For this review, take the finished solid that the model builds, in its own axes (mm). Face numbers are marked on the shaded views. A direction names the side the tool comes from. Coordinates: 2 decimals unless noted, no trailing zeros. Order: outer loops, then holes, each group sorted by start corner. A loop starts at its lowest first (then second) coordinate and runs counter-clockwise, first axis right, second up. Notation, with made-up numbers: (58.5, 53.5) -> (88.5, 53.5) arc R16 cw to (88.5, 84.5) -> close; hole circle Ø11 at (-6.5, 75.5). An arc over 180 degrees is marked (long way). Write item = value, one per line. Start each with the question number.
1) Machinability: for the marked faces 1 and 2, which of the approach directions +Z, -Z, +X, -X, +Y, -Y give a long, thin tool a straight path to every point of the face, cutting with its end or side? Answer none if there is none.
2) Draft analysis for pull direction X (two halves, no side actions). For the marked faces 3, 4 and 5, state which applies: +X half, -X half, draft (parallel to the pull), parting line (faces both ways), or undercut.
3) Insertion check: pin 1 Ø6 at (x, z) = (-79, 7.5) entering from -Y; pin 2 Ø4 at (x, z) = (-54, 30) entering from +Y; pin 3 Ø6 at (y, z) = (10, 43) entering from -X; pin 4 Ø5 at (x, y) = (31, 14.5) entering from -Z. Each pin has a flat end and moves straight along its axis. Give the tip position at first contact, or say it passes through.
4) Wall thickness on probe 1 along Y at (x, z) = (-70, 32.5); probe 2 along Z at (x, y) = (-20.5, 45.5); probe 3 along X at (y, z) = (2, 4): over which ranges is each line inside the solid? List them lowest first. Write a range as [from, to].
5) Consider section A-A on x = 54. Give the boundary of the cut face in (y, z).
6) Consider section D-D on y = -23. Give the boundary of the cut face in (x, z), and give its area (3 significant figures).
7) Consider section C-C on z = 4.5. Give the boundary of the cut face in (x, y).
8) Consider section B-B on y = -10. Give the boundary of the cut face in (x, z), and give its area (3 significant figures).
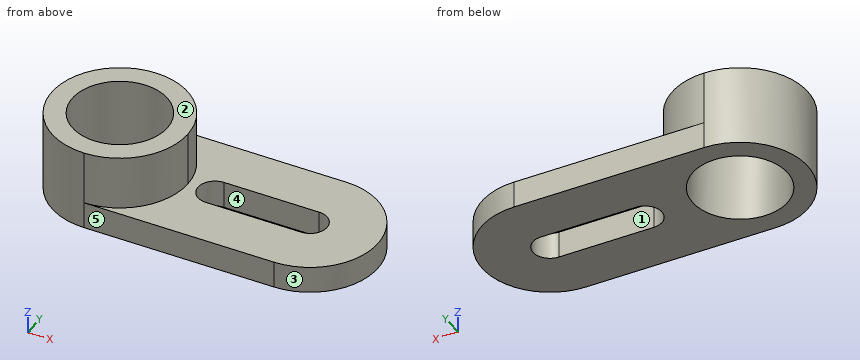
from build123d import *

# Parameters (mm, degrees)
F0_R     = 35
F1_DEPTH = 20
F2_DEPTH = 60


with BuildPart() as f1:
    # F0 (on Top) → F1 (new body)
    with BuildSketch(Plane.XY):
        with BuildLine():
            ThreePointArc((-70, -50), (-34.644661, -35.355339), (-20, 0))
            ThreePointArc((-20, 0), (-34.644661, 35.355339), (-70, 50))
            ThreePointArc((-70, 50), (-120, 0), (-70, -50))
        make_face()
        with Locations((-70, 0)):
            Circle(F0_R, mode=Mode.SUBTRACT)
        with BuildLine():
            ThreePointArc((-70, 50), (-34.644661, 35.355339), (-20, 0))
            ThreePointArc((-20, 0), (-34.644661, -35.355339), (-70, -50))
            Line((-70, -50), (70, -50))
            ThreePointArc((70, -50), (120, 0), (70, 50))
            Line((70, 50), (-70, 50))
        make_face()
        with BuildLine():
            Line((70, -12.5), (0, -12.5))
            ThreePointArc((0, -12.5), (-12.5, 0), (0, 12.5))
            Line((0, 12.5), (70, 12.5))
            ThreePointArc((70, 12.5), (82.5, 0), (70, -12.5))
        make_face(mode=Mode.SUBTRACT)
    extrude(amount=F1_DEPTH)

    # F0 (on Top) → F2 (join)
    with BuildSketch(Plane.XY):
        with BuildLine():
            ThreePointArc((-70, -50), (-34.644661, -35.355339), (-20, 0))
            ThreePointArc((-20, 0), (-34.644661, 35.355339), (-70, 50))
            ThreePointArc((-70, 50), (-120, 0), (-70, -50))
        make_face()
        with Locations((-70, 0)):
            Circle(F0_R, mode=Mode.SUBTRACT)
    extrude(amount=F2_DEPTH)


solid = f1.part
Answer sheet:
q1.face_1 = +Z, -Z
q1.face_2 = +Z, +X, -X, +Y, -Y
q2.face_3 = +X half
q2.face_4 = undercut
q2.face_5 = draft
q3.pin_1 = -49.64
q3.pin_2 = 48
q3.pin_3 = -119.51
q3.pin_4 = 0
q4.probe_1 = [-50, -35], [35, 50]
q4.probe_2 = [0, 20]
q4.probe_3 = [-119.96, -104.94], [-35.06, -12.34], [82.34, 119.96]
q5.outline = (-50, 0) -> (-12.5, 0) -> (-12.5, 20) -> (-50, 20) -> close; (12.5, 0) -> (50, 0) -> (50, 20) -> (12.5, 20) -> close
q6.outline = (-114.4, 0) -> (-96.38, 0) -> (-96.38, 60) -> (-114.4, 60) -> close; (-43.62, 0) -> (114.4, 0) -> (114.4, 20) -> (-25.6, 20) -> (-25.6, 60) -> (-43.62, 60) -> close
q6.area = 4,960 mm2
q7.outline = (-70, -50) -> (70, -50) arc R50 ccw to (70, 50) -> (-70, 50) arc R50 ccw to start; hole circle Ø70 at (-70, 0); hole (0, -12.5) -> (70, -12.5) arc R12.5 ccw to (70, 12.5) -> (0, 12.5) arc R12.5 ccw to start
q8.outline = (-118.99, 0) -> (-103.54, 0) -> (-103.54, 60) -> (-118.99, 60) -> close; (-36.46, 0) -> (-7.5, 0) -> (-7.5, 20) -> (-21.01, 20) -> (-21.01, 60) -> (-36.46, 60) -> close; (77.5, 0) -> (118.99, 0) -> (118.99, 20) -> (77.5, 20) -> close
q8.area = 2,950 mm2
